Autodesk Inventor part; units mm, degrees
ref_plane "YZ Plane" through (0, 0, 0) normal (1, 0, 0) x (0, 1, 0)
ref_plane "XZ Plane" through (0, 0, 0) normal (0, 1, 0) x (-1, 0, 0)
ref_plane "XY Plane" through (0, 0, 0) normal (0, 0, 1) x (1, 0, 0)
sketch "Sketch1" plane through (0, 0, 0) normal (0, 0, 1) x (1, 0, 0)
  line L0 (0, 0) -> (38.1, 0)
  line L1 (38.1, 0) -> (38.1, 22.86)
  line L2 (38.1, 22.86) -> (0, 22.86)
  line L3 (0, 22.86) -> (0, 0)
  dimension "d0" = 22.86
  dimension "d1" = 38.1
extrude "Extrusion1" add sketch "Sketch1" along normal blind 2.54
sketch "Sketch2" plane through (0, 0, 2.54) normal (0, 0, 1) x (1, 0, 0)
  line L0 (0, 0) -> (38.1, 0)
  line L1 (38.1, 22.86) -> (35.56, 22.86)
  line L2 (35.56, 22.86) -> (35.56, 0)
  line L3 (35.56, 0) -> (38.1, 0)
  line L4 (38.1, 0) -> (38.1, 22.86)
  dimension "d4" = 2.54
extrude "Extrusion2" add sketch "Sketch2" along normal blind 35.56
sketch "Sketch4" plane through (0, 0, 2.54) normal (0, 0, 1) x (1, 0, 0)
  line L0 (-11.3987, 11.43) -> (43.7828, 11.43) construction
  line L1 (0, 0) -> (35.56, 0) construction
  line L2 (35.56, 0) -> (35.56, 22.86) construction
  line L3 (35.56, 22.86) -> (0, 22.86) construction
  line L4 (0, 22.86) -> (0, 0) construction
  line L5 (0, 0) -> (35.56, 0) construction
  point P0 (10.16, 11.43)
  dimension "d16" = 11.43
  dimension "d17" = 25.4
hole "Hole2" at (10.16, 11.43, 2.54) direction (0, 0, -1) diameter 3.2512 end through all
sketch "Sketch5" plane through (35.56, 0, 2.54) normal (-1, 0, 0) x (0, 0, 1)
  line L0 (25.4046, 11.4617) -> (26.6746, 11.4617)
  circle A0 centre (26.6746, 11.4617) radius 1.6412
  point P0 (-2.54, 0)
  dimension "d25" = 1.27
extrude "Extrusion3" cut sketch "Sketch5" against normal blind 25.4
properties part number "000102 (revised)"
Here's how the part is built. I have some questions about the finished solid (model axes, mm). A direction names the side the tool comes from. Coordinates: 2 decimals unless noted, no trailing zeros. Order: outer loops, then holes, each group sorted by start corner. A loop starts at its lowest first (then second) coordinate and runs counter-clockwise, first axis right, second up. Notation, with made-up numbers: (-16.75, 80.25) -> (7.25, 80.25) arc R16 ccw to (7.25, 93.25) -> close; hole circle Ø10 at (33, 56). An arc over 180 degrees is marked (long way). Return JSON: item names as keys, results as strings.
1) If we section it at B-B on y = 14.25: List the corners of the cut face in (x, z) for me, plus the area to 3 significant figures.
Conclusion:
{"outline": "(0, 0) -> (38.1, 0) -> (38.1, 38.1) -> (35.56, 38.1) -> (35.56, 2.54) -> (0, 2.54) -> close", "area": "187 mm²"}
2) If I drill on probe 1 along X at (y, z) = (11.43, 1.05); probe 2 along X at (y, z) = (6.75, 20); probe 3 along Z at (x, y) = (12, 21.5), over which ranges is the centre line in solid material (lowest first)?
Conclusion:
{"probe 1": "x = 0 to 8.53, 11.79 to 38.1", "probe 2": "x = 35.56 to 38.1", "probe 3": "z = 0 to 2.54"}
3) On a 3-axis mill with a long thin cutter (end or side, diameter ignored), from which of +Z, -Z, +X, -X, +Y, -Y can I reach the whole of each face in a straight line? I mean faces 1 (the cylindrical face through (36.81, 11.95, 30.78)), 2 (the flat face through (18, 12, 2.54)). Say none if no direction works.
Conclusion:
{"face 1": "+X, -X", "face 2": "+Z, -X, +Y, -Y"}
4) If we section it at A-A on x = 10.16: List the corners of the cut face in (y, z) for me, plus the area to 3 significant figures.
Conclusion:
{"outline": "(0, 0) -> (9.8, 0) -> (9.8, 2.54) -> (0, 2.54) -> close; (13.06, 0) -> (22.86, 0) -> (22.86, 2.54) -> (13.06, 2.54) -> close", "area": "49.8 mm²"}
5) If we section it at D-D on z = 27: List the corners of the cut face in (x, y) for me.
Conclusion:
{"outline": "(35.56, 0) -> (38.1, 0) -> (38.1, 22.86) -> (35.56, 22.86) -> close"}
6) If we section it at C-C on x = 19: List the corners of the cut face in (y, z) for me.
Conclusion:
{"outline": "(0, 0) -> (22.86, 0) -> (22.86, 2.54) -> (0, 2.54) -> close"}
7) I'm going to push flat-ended pins straight in: P1, Ø5.5, axis at y = 11.46, z = 29.21, coming from the -X side; P2, Ø8, axis at x = 24.5, y = 17, coming from the +Z side; P3, Ø1, axis at x = 9.5, y = 20, coming from the -Z side; P4, Ø10, axis at x = 17, z = 11, coming from the -Y side. Where does each tip first touch, or does it pass through?
Conclusion:
{"P1": "stops at x = 35.56", "P2": "stops at z = 2.54", "P3": "stops at z = 0", "P4": "passes through"}
8) Thinking about a two-plate mould opening in X: for faces 3 (the cylindrical face through (8.55, 11.64, 1.25)), 4 (the flat face through (35.56, 12, 20)), 5 (the flat face through (36, 22.86, 10)), which applies, +X half, -X half, draft (parallel to the pull), parting line (faces both ways), or undercut?
Conclusion:
{"face 3": "undercut", "face 4": "-X half", "face 5": "draft"}
